Build history of the part. All positions in model axes, mm. Face numbers are marked on the shaded views. Round coordinates to 2 decimals unless told otherwise and drop trailing zeros. Loops run counter-clockwise (first coordinate to the right, second up) from the corner with the lowest first, then second, coordinate; pieces in that order, holes last. Notation, with made-up numbers: (8.25, 27.25) -> (64.25, 27.25) arc R22 ccw to (64.25, 65.25) -> close; hole circle Ø6 at (-36, 20). An arc over 180 degrees is marked (long way). Put each result on its own line as item: value. Start each with the question number.
```python
from build123d import *

# Parameters (mm, degrees)
BOSS_EXTRUDE1_DEPTH = 19.05
SKETCH2_R           = 3.96875
CUT_EXTRUDE1_DEPTH  = 19.05
SKETCH3_W           = 457.2
SKETCH3_H           = 152.4
BOSS_EXTRUDE3_DEPTH = 19.05
SKETCH4_W           = 457.2
SKETCH4_H           = 152.4
CUT_EXTRUDE2_DEPTH  = 25.4
CUT_EXTRUDE4_DEPTH  = 25.4
SKETCH6_W           = 457.2
SKETCH6_H           = 152.4
BOSS_EXTRUDE4_DEPTH = 3.175


with BuildPart() as part:
    # Sketch1 → Boss-Extrude1 (new body)
    with BuildSketch(Plane(origin=(0, 0, 0), x_dir=(1, 0, 0), z_dir=(0, 1, 0))):
        Polygon((57.15, 19.05), (0, 19.05), (0, 0), (66.037825848, 0), (97.808358016, 38.1), (336.311308439, 38.1), (400.965853894, -12.7), (431.8, -12.7), (342.9, 57.15), (88.9, 57.15), align=None)
    extrude(amount=BOSS_EXTRUDE1_DEPTH)

    # Sketch2 → Cut-Extrude1 (cut)
    with BuildSketch(Plane.XY):
        with Locations((8.89, 9.525)):
            Circle(SKETCH2_R)
        with Locations((56.515, 9.525)):
            Circle(SKETCH2_R)
    extrude(amount=-CUT_EXTRUDE1_DEPTH, mode=Mode.SUBTRACT)

    # Sketch4 → Cut-Extrude2 (cut)
    with BuildSketch(Plane(origin=(0, 0, 0), x_dir=(1, 0, 0), z_dir=(0, 1, 0))):
        with Locations((215.9, 38.1)):
            Rectangle(SKETCH4_W, SKETCH4_H)
    extrude(amount=CUT_EXTRUDE2_DEPTH, mode=Mode.SUBTRACT)


with BuildPart() as body_2:
    # Sketch3 → Boss-Extrude3 (new body)
    with BuildSketch(Plane.XZ):
        with Locations((215.9, -38.1)):
            Rectangle(SKETCH3_W, SKETCH3_H)
        Polygon((400.965853894, 12.7), (431.8, 12.7), (342.9, -57.15), (88.9, -57.15), (57.15, -19.05), (0, -19.05), (0, 0), (66.037825848, 0), (97.808358016, -38.1), (336.311308439, -38.1), align=None, mode=Mode.SUBTRACT)
    extrude(amount=BOSS_EXTRUDE3_DEPTH)

    # Sketch5 → Cut-Extrude4 (cut)
    with BuildSketch(Plane.XZ.offset(19.05)):
        Polygon((-12.7, -19.05), (0, -19.05), (0, 0), (66.037825848, 0), (97.808358016, -38.1), (336.311308439, -38.1), (400.965853894, 12.7), (431.8, 12.7), (431.8, 38.1), (-12.7, 38.1), align=None)
    extrude(amount=-CUT_EXTRUDE4_DEPTH, mode=Mode.SUBTRACT)

    # Sketch6 → Boss-Extrude4 (add)
    with BuildSketch(Plane(origin=(0, 0, 0), x_dir=(1, 0, 0), z_dir=(0, 1, 0))):
        with Locations((215.9, 38.1)):
            Rectangle(SKETCH6_W, SKETCH6_H)
    extrude(amount=BOSS_EXTRUDE4_DEPTH)


solid = body_2.part
```
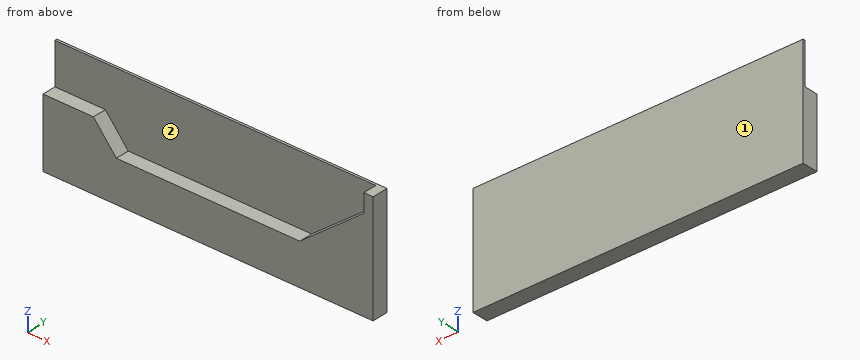
Item 1: Cut at D-D on z = -47. Write the cut outline in (x, y) (3 decimals), then the cut area to 3 significant figures.
Item 2: Pull direction X, two halves, no side cores. Call the marked faces 1 and 2: +X half, -X half, draft (parallel to the pull), parting line (faces both ways), or undercut.
Item 3: Cut at B-B on x = 312.5. Write the cut outline in (y, z) (3 decimals).
Item 4: Wall check: line 1 (Y direction, x = 172, z = -55.5) (3 decimals); line 2 (X direction, y = -7, z = 32.5); line 3 (X direction, y = -12, z = -22). Give the ranges that are in metal, low to high. Write a range as from..to.
Item 5: Drop flat-ended pins along their axis: pin 1 (9.5 mm diameter, centred on x = 182, y = -5.5, fed in from +Z); pin 2 (5 mm diameter, centred on y = -3, z = -6.5, fed in from -X); pin 3 (3 mm diameter, centred on x = 81.5, y = -15, fed in from +Z). Give the stop position or say it passes through.
Item 6: Cut at A-A on y = -8.5. Write the cut outline in (x, z).
Item 7: Cut at C-C on z = 20. Write the cut outline in (x, y) (3 decimals), then the cut area to 3 significant figures.
Ans:
1. outline: (-12.7, -19.05) -> (80.442, -19.05) -> (80.442, 0) -> (355.818, 0) -> (355.818, -19.05) -> (444.5, -19.05) -> (444.5, 3.175) -> (-12.7, 3.175) -> close
1. area: 4,920 mm2
2. face 1: draft
2. face 2: undercut
3. outline: (-19.05, -114.3) -> (3.175, -114.3) -> (3.175, 38.1) -> (0, 38.1) -> (0, -57.15) -> (-19.05, -57.15) -> close
4. line 1: y = 0..3.175
4. line 2: x = 431.8..444.5
4. line 3: x = -12.7..59.61, 387.64..444.5
5. pin 1: stops at z = -57.15
5. pin 2: stops at x = 404.18
5. pin 3: stops at z = -46.47
6. outline: (-12.7, -114.3) -> (444.5, -114.3) -> (444.5, 38.1) -> (431.8, 38.1) -> (431.8, 12.7) -> (342.9, -57.15) -> (88.9, -57.15) -> (57.15, -19.05) -> (-12.7, -19.05) -> close
7. outline: (-12.7, 0) -> (431.8, 0) -> (431.8, -19.05) -> (444.5, -19.05) -> (444.5, 3.175) -> (-12.7, 3.175) -> close
7. area: 1,690 mm2
